Autodesk Inventor part; units mm, degrees
ref_plane "Płaszczyzna konstrukcyjna1" through (16.1843, 0, -20) normal (-1, 0, 0) x (0, 0, 1)
ref_plane "Płaszczyzna konstrukcyjna2" through (25.1843, 0, -20) normal (1, 0, 0) x (0, 1, 0)
ref_plane "Płaszczyzna konstrukcyjna3" through (-5.8487, 1.5, -21) normal (0, 0, 1) x (1, 0, 0)
sketch "Szkic1" plane through (0, 0, 0) normal (1, 0, 0) x (0, 1, 0)
  line L0 (0, 0) -> (12, 0)
  line L1 (12, 0) -> (12, -10)
  line L2 (16, -10) -> (16, 4)
  line L3 (16, 4) -> (0, 4)
  line L4 (0, 4) -> (0, 0)
  line L5 (12, -10) -> (16, -10)
  dimension "d0" = 12
  dimension "d1" = 10
  dimension "d2" = 4
extrude "Wyciągnięcie proste1" add sketch "Szkic1" along normal blind 9
sketch "Szkic2" plane through (0, 0, 0) normal (-1, 0, 0) x (0, 0, 1)
  arc A0 (-10.2, 9.6) -> (-19.8, 9.6) centre (-15, 6) ccw
  line L0 (-10, 12) -> (-10, 16)
  line L1 (-10, 12) -> (-10.2, 12)
  line L2 (-10.2, 12) -> (-10.2, 9.6)
  line L3 (-10, 11) -> (-10, 1)
  line L4 (-10, 11) -> (-10, 12)
  line L5 (-10.2, 9.6) -> (-10, 9.3166)
  line L6 (-19.8, 9.6) -> (-19.8, 16)
  line L7 (-10, 16) -> (4, 16)
  line L8 (-19.8, 16) -> (-10, 16)
  point P0 (0, 0)
extrude "Wyciągnięcie proste2" add sketch "Szkic2" against normal up to surface (9 mm away)
sketch "Szkic3" plane through (9, 0, 0) normal (1, 0, 0) x (0, 0, -1)
  line L0 (0, 12) -> (10, 12)
  line L1 (10, 9.3166) -> (10, 12)
  line L2 (10.2, 9.6) -> (10, 9.3166)
  arc A0 (19.8, 9.6) -> (10.2, 9.6) centre (15, 6) ccw
  line L3 (19.8, 16) -> (19.8, 9.6)
  line L4 (-4, 16) -> (19.8, 16)
  line L5 (-4, 16) -> (-4, 0)
  line L6 (-4, 0) -> (0, 0)
  line L7 (0, 0) -> (0, 12)
  arc A1 (9.8, 9.6) -> (0.2, 9.6) centre (5, 6) ccw
  line L8 (9.8, 9.6) -> (10, 9.3166)
  line L9 (0.2, 9.6) -> (0, 9.3166)
ref_plane "Płaszczyzna konstrukcyjna1" through (16.1843, 0, -20) normal (-1, 0, 0) x (0, 0, 1)
extrude "Wyciągnięcie proste3" add sketch "Szkic3" along normal up to surface (7.1843 mm away)
sketch "Szkic4" plane through (16.1843, 0, 4) normal (1, 0, 0) x (0, 0, -1)
  line L0 (23, 12) -> (15, 12)
  arc A0 (13.8, 9.6) -> (4.2, 9.6) centre (9, 6) ccw
  line L1 (13.8, 9.6) -> (14, 9.3166)
  line L2 (14, 9.3166) -> (14.2, 9.6)
  arc A1 (23.8, 9.6) -> (14.2, 9.6) centre (19, 6) ccw
  line L3 (23.8, 9.6) -> (23.8, 16)
  line L4 (23.8, 16) -> (0, 16)
  line L5 (0, 16) -> (0, 0)
  line L6 (0, 0) -> (4, 0)
  line L7 (4, 0) -> (4, 9.3166)
  line L8 (4, 9.3166) -> (4.2, 9.6)
  line L9 (23, 12) -> (23.8, 12)
  line L10 (23.8, 9.6) -> (23.8, 16)
  line L11 (14, 11) -> (14, 1)
  line L12 (15, 12) -> (14, 12)
  line L13 (14, 12) -> (14, 11)
  point P0 (4, 0)
ref_plane "Płaszczyzna konstrukcyjna2" through (25.1843, 0, -20) normal (1, 0, 0) x (0, 1, 0)
extrude "Wyciągnięcie proste4" add sketch "Szkic4" along normal up to surface (9 mm away) contours L0 L12 L13 L11 L1 A0 L8 L7 L6 L5 L4 L3 L9
sketch "Szkic5" plane through (0, 9.6, -19.8) normal (0, 0, -1) x (-1, 0, 0)
  line L0 (0, 0) -> (-16.1843, 0)
  line L1 (0, 6.4) -> (0, 0)
  line L2 (0, 6.4) -> (-25.1843, 6.4)
  line L3 (-25.1843, 6.4) -> (-25.1843, 2.4)
  line L4 (-16.1843, 2.4) -> (-25.1843, 2.4)
  line L5 (-16.1843, 0) -> (-16.1843, 2.4)
  line L6 (0, -9.6) -> (-25.1843, -9.6)
  line L7 (0, 6.4) -> (-25.1843, 6.4)
  line L8 (-25.1843, 6.4) -> (0, 6.4)
  line L9 (0, 6.4) -> (0, -9.6)
  line L10 (0, -9.6) -> (-25.1843, -9.6)
  line L11 (-25.1843, -9.6) -> (-25.1843, 6.4)
ref_plane "Płaszczyzna konstrukcyjna3" through (-5.8487, 1.5, -21) normal (0, 0, 1) x (1, 0, 0)
extrude "Wyciągnięcie proste5" add sketch "Szkic5" along normal up to surface (1.2 mm away)
sketch "Szkic6" plane through (0, 0, -19.8) normal (0, -1, 0) x (1, 0, 0)
  line L0 (32.6513, -1.7) -> (32.6513, -14.7)
  line L1 (32.1513, -15.2) -> (-5.8487, -15.2)
  line L2 (-5.8487, -1.2) -> (32.1513, -1.2)
  line L3 (-6.3487, -14.7) -> (-6.3487, -1.7)
  line L4 (32.6513, -1.2) -> (-6.3487, -1.2)
  line L5 (-6.3487, -1.2) -> (-6.3487, -15.2)
  line L6 (-6.3487, -15.2) -> (32.6513, -15.2)
  line L7 (32.6513, -15.2) -> (32.6513, -1.2)
  line L8 (-6.5487, -1) -> (32.8513, -1)
  line L9 (32.8513, -1) -> (32.8513, -15.4)
  line L10 (32.8513, -15.4) -> (-6.5487, -15.4)
  line L11 (-6.5487, -15.4) -> (-6.5487, -1)
  line L12 (34.8513, 1) -> (-8.5487, 1)
  line L13 (-8.5487, 1) -> (-8.5487, -17.4)
  line L14 (-8.5487, -17.4) -> (34.8513, -17.4)
  line L15 (34.8513, -17.4) -> (34.8513, 1)
  line L16 (16.1843, 0) -> (25.1843, 0)
  line L17 (25.1843, 0) -> (25.1843, -1.2)
  line L18 (25.1843, 0) -> (34.8513, 0)
  line L19 (32.8513, -1) -> (32.8513, 1)
  line L20 (25.1843, 0) -> (0, 0)
  line L21 (0, 0) -> (-8.5487, 0)
  line L22 (-6.5487, -1) -> (-6.5487, 1)
  point P0 (0, 19.8)
  dimension "d13" = 0.2
  dimension "d14" = 2
extrude "Wyciągnięcie proste6" add sketch "Szkic6" against normal blind 1 contours L8 L9 L10 L11 | L8 L22 L21 L20 L16 L17 | L17 L18 L19 L8 | L0 L7 L6 L1 L5 L3 L4 L2 | L11 L10 L9 L19 L18 L15 L14 L13 L21 L22
sketch "Szkic7" plane through (0, 1, -19.8) normal (0, 1, 0) x (1, 0, 0)
  line L0 (0, 1.2) -> (0, 0)
  line L1 (25.1843, 1.2) -> (0, 1.2)
  line L2 (25.1843, 0) -> (25.1843, 1.2)
  line L3 (25.1843, 0) -> (34.8513, 0)
  line L4 (34.8513, 0) -> (34.8513, 17.4)
  line L5 (34.8513, 17.4) -> (-8.5487, 17.4)
  line L6 (-8.5487, 17.4) -> (-8.5487, 0)
  line L7 (-8.5487, 0) -> (0, 0)
  line L8 (32.8513, 15.4) -> (32.8513, 2)
  line L9 (-2, 2) -> (-6.5487, 2)
  line L10 (-6.5487, 2) -> (-6.5487, 15.4)
  line L11 (-6.5487, 15.4) -> (32.8513, 15.4)
  line L12 (0, 1.2) -> (-6.5487, 2)
  line L13 (32.8513, 2) -> (34.8513, 2)
  line L14 (34.8513, 0) -> (34.8513, 17.4)
  point P0 (0, -19.8)
  point P1 (34.8513, 2)
  dimension "d17" = 2
extrude "Wyciągnięcie proste7" add sketch "Szkic7" along normal blind 8 contours L0 L7 L6 L5 L4 L13 L8 L11 L10 L12
fillet "Zaokrąglenie1" radius 2 3 edges at (34.8513, 4.5, -37.2) (-8.5487, 4.5, -37.2) (-8.5487, 4.5, -19.8)
sketch "Szkic8" plane through (25.1843, 0, 4) normal (1, 0, 0) x (0, 0, -1)
  line L0 (23.8, 1) -> (25, 1)
  line L1 (25, 16) -> (25, 1)
  line L2 (0, 16) -> (25, 16)
  line L3 (0, 0) -> (0, 16)
  line L4 (4, 0) -> (0, 0)
  line L5 (4, 9.3166) -> (4, 0)
  line L6 (4.2, 9.6) -> (4, 9.3166)
  arc A0 (13.8, 9.6) -> (4.2, 9.6) centre (9, 6) ccw
  line L7 (14, 9.3166) -> (13.8, 9.6)
  line L8 (14, 12) -> (14, 9.3166)
  line L9 (23.8, 12) -> (14, 12)
  line L10 (23.8, 12) -> (23.8, 1)
  line L11 (23.8, 12) -> (14, 12)
  line L12 (14, 12) -> (14, 16)
  line L13 (0, 16) -> (25, 16)
  point P0 (4, 0)
  point P1 (14, 16)
ref_plane "Płaszczyzna konstrukcyjna4" through (27.1843, 3.25, -7.75) normal (1, 0, 0) x (0, 1, 0)
extrude "Wyciągnięcie proste8" add sketch "Szkic8" along normal up to surface (2 mm away) contours L8 L7 A0 L6 L5 L4 L3 L2 L12
sketch "Szkic9" plane through (27.1843, 0, 4) normal (1, 0, 0) x (0, 0, -1)
  circle A0 centre (9, 6) radius 2.75
  arc A1 (13.8, 9.6) -> (4.2, 9.6) centre (9, 6) ccw
  line L0 (14, 9.3166) -> (14, 0)
  line L1 (4, 9.3166) -> (4, 0)
  line L2 (4.2, 9.6) -> (4, 9.3166)
  line L3 (4, 0) -> (14, 0)
  line L4 (14, 9.3166) -> (13.8, 9.6)
extrude "Wyciągnięcie proste9" add sketch "Szkic9" against normal blind 0.8
sketch "Szkic10" plane through (27.1843, 0, 4) normal (1, 0, 0) x (0, 0, -1)
  circle A0 centre (9, 6) radius 1.47
  circle A1 centre (9, 6) radius 2.75
  line L0 (0, 0) -> (0, 16)
  line L1 (0, 0) -> (14, 0)
  line L2 (14, 16) -> (14, 0)
  line L3 (0, 16) -> (14, 16)
  point P0 (4, 0)
extrude "Wyciągnięcie proste10" add sketch "Szkic10" along normal blind 3.2 contours A1 | L0 L3 L2 L1
sketch "Szkic11" plane through (26.3843, 0, 4) normal (-1, 0, 0) x (0, 0, 1)
  circle A0 centre (-9, 6) radius 2.75
  circle A1 centre (-9, 6) radius 2.95
  point P0 (-4, 0)
  dimension "d27" = 0.2
extrude "Wyciągnięcie proste11" cut sketch "Szkic11" against normal up to surface (0.8 mm away) contours A0 | A1
sketch "Szkic12" plane through (27.1843, 6, -5) normal (-1, 0, 0) x (0, 0, 1)
  circle A0 centre (0, 0) radius 1.47
  circle A1 centre (0, 0) radius 1.67
  point P0 (5, -6)
  dimension "d30" = 0.2
extrude "Wyciągnięcie proste12" cut sketch "Szkic12" against normal through all contours A0 | A1
properties part number "montaz_silniki"
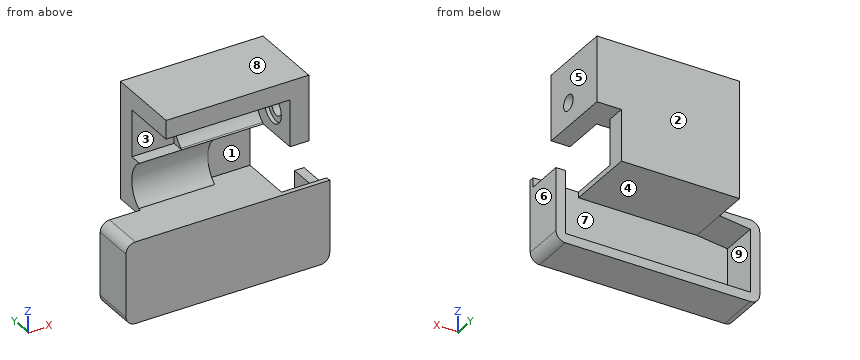
Verification items for the finished model (mm, model axes). Face numbers are marked on the shaded views. A direction names the side the tool comes from. Give positions to 0.01 mm unless a question says otherwise; leave off trailing zeros. Write each loop counter-clockwise with the first axis right and the second up, starting at its lowest first coordinate (ties: lowest second). Pieces come first, ordered by that corner, then holes. Notation, with made-up numbers: M 20.5,-11 L 55.5,-11 A7 ccw 55.5,-7 Z; hole C 16,-37 d1. An arc over 180 degrees is marked long. Put each result on its own line as item: value. Start each with the question number.
1. Scan lines: line 1 along Y through (x, z) = (27.95, -5); line 2 along X through (y, z) = (7.5, -31.5); line 3 along Z through (x, y) = (5.5, 1.5). Record each from-to range of solid material in increasing order. Write a range as [from, to].
2. Section check B-B (y = 6). Record the cut outline in (x, z).
3. Section check C-C (x = 19). Record the cut outline in (y, z).
4. Draft check along X on the marked faces 6, 7, 8 and 9. Enter one of: +X half, -X half, draft (parallel to the pull), parting line (faces both ways), or undercut.
5. Go/stop test with flat-tipped pins: pin 1 Ø5 at (y, z) = (7.5, -0.5) entering from +X; pin 2 Ø1.3 at (y, z) = (10.5, -7) entering from -X; pin 3 Ø8 at (y, z) = (8, -2.5) entering from -X. Record where each tip stops, or that it passes through.
6. Section check D-D (z = -26). Record the cut outline in (x, y).
7. Section check A-A (y = 1.5). Record the cut outline in (x, z).
8. Set-up check for the marked faces 1, 2, 3, 4 and 5: record each of +Z, -Z, +X, -X, +Y, -Y from which the full face is reachable in a straight line by a thin tool's end or side.
Answer list:
1. line 1: [0, 4.33], [7.67, 16]
1. line 2: [-8.55, -6.55], [32.85, 34.85]
1. line 3: [-37.2, -35.2], [-21, -19.8], [0, 4]
2. outline: M -8.55,-35.2 A2 ccw -6.55,-37.2 L 32.85,-37.2 A2 ccw 34.85,-35.2 L 34.85,-21.8 L 32.85,-21.8 L 32.85,-35.2 L -6.55,-35.2 L -6.55,-21.8 L 0,-21 L 25.18,-21 L 25.18,-19.8 L -6.55,-19.8 A2 ccw -8.55,-21.8 Z; M 0,0 L 26.38,0 L 26.38,-2.05 L 27.18,-2.05 L 27.18,-3.33 L 30.38,-3.33 L 30.38,4 L 0,4 Z; M 26.38,-10 L 30.38,-10 L 30.38,-6.67 L 27.18,-6.67 L 27.18,-7.95 L 26.38,-7.95 Z
3. outline: M 0,-37.2 L 9,-37.2 L 9,-35.2 L 1,-35.2 L 1,-21 L 16,-21 L 16,4 L 0,4 L 0,0 L 9.32,0 L 9.6,-0.2 A6 cw 9.6,-9.8 L 9.32,-10 L 12,-10 L 12,-19.8 L 0,-19.8 Z
4. face 6: +X half
4. face 7: undercut
4. face 8: draft
4. face 9: undercut
5. pin 1: x = 30.38
5. pin 2: x = 26.38
5. pin 3: x = 0
6. outline: M -8.55,0 L 34.85,0 L 34.85,9 L 32.85,9 L 32.85,1 L -6.55,1 L -6.55,9 L -8.55,9 Z
7. outline: M -8.55,-35.2 A2 ccw -6.55,-37.2 L 32.85,-37.2 A2 ccw 34.85,-35.2 L 34.85,-21.8 L 32.85,-21.8 L 32.85,-35.2 L -6.55,-35.2 L -6.55,-21.8 L 0,-21 L 25.18,-21 L 25.18,-19.8 L -6.55,-19.8 A2 ccw -8.55,-21.8 Z; M 0,0 L 26.38,0 L 26.38,-10 L 30.38,-10 L 30.38,4 L 0,4 Z
8. face 1: +X, -Y
8. face 2: +Z, -Z, +X, -X, +Y
8. face 3: -X, -Y
8. face 4: +X, +Y
8. face 5: +Z, +X, +Y, -Y
